from build123d import *

# Parameters (mm, degrees)
SKETCH1_R               = 12.7
EXTRUDE1_DEPTH          = 76.2
SKETCH2_R               = 5
EXTRUDE2_DEPTH          = 2
SKETCH3_R               = 13.7
EXTRUDE3_DEPTH          = 4
SKETCH4_R               = 4
EXTRUDE4_DEPTH          = 7
SKETCH5_W               = 279.527972269
SKETCH5_H               = 9.602426348
CUT_EXTRUDE1_DEPTH      = 14.7
CUT_EXTRUDE1_DEPTH_BACK = 14.7


with BuildPart() as part:
    # Sketch1 → Extrude1 (new body)
    with BuildSketch(Plane(origin=(0, 0, 0), x_dir=(0, 0, -1), z_dir=(1, 0, 0))):
        Circle(SKETCH1_R)
    extrude(amount=EXTRUDE1_DEPTH)

    # Sketch2 → Extrude2 (add, symmetric)
    with BuildSketch(Plane.XY):
        with BuildLine():
            Line((0, 9.805687548), (-19.733094472, 9.805687548))
            ThreePointArc((-19.733094472, 9.805687548), (-29.53878202, 0), (-19.733094472, -9.805687548))
            Line((-19.733094472, -9.805687548), (0, -9.805687548))
            Line((0, -9.805687548), (0, 9.805687548))
        make_face()
        with Locations((-19.733094472, 0)):
            Circle(SKETCH2_R, mode=Mode.SUBTRACT)
    extrude(amount=EXTRUDE2_DEPTH, both=True)

    # Sketch3 → Extrude3 (add)
    with BuildSketch(Plane(origin=(76.2, 0, 0), x_dir=(0, 0, -1), z_dir=(1, 0, 0))):
        Circle(SKETCH3_R)
    extrude(amount=EXTRUDE3_DEPTH)

    # Sketch4 → Extrude4 (add, symmetric)
    with BuildSketch(Plane.XY):
        with BuildLine():
            Line((80.2, 9.635666442), (106.2, 9.635666442))
            ThreePointArc((106.2, 9.635666442), (115.835666442, 0), (106.2, -9.635666442))
            Line((106.2, -9.635666442), (80.2, -9.635666442))
            Line((80.2, -9.635666442), (80.2, 9.635666442))
        make_face()
        with Locations((106.2, 0)):
            Circle(SKETCH4_R, mode=Mode.SUBTRACT)
    extrude(amount=EXTRUDE4_DEPTH, both=True)

    # Sketch5 → Cut-Extrude1 (cut, two sides)
    with BuildSketch(Plane(origin=(0, 0, 0), x_dir=(1, 0, 0), z_dir=(0, 1, 0))) as cut_extrude1_sk:
        with Locations((219.963986135, 0)):
            Rectangle(SKETCH5_W, SKETCH5_H)
    extrude(amount=CUT_EXTRUDE1_DEPTH, mode=Mode.SUBTRACT)
    extrude(cut_extrude1_sk.sketch, amount=-CUT_EXTRUDE1_DEPTH_BACK, mode=Mode.SUBTRACT)


solid = part.part
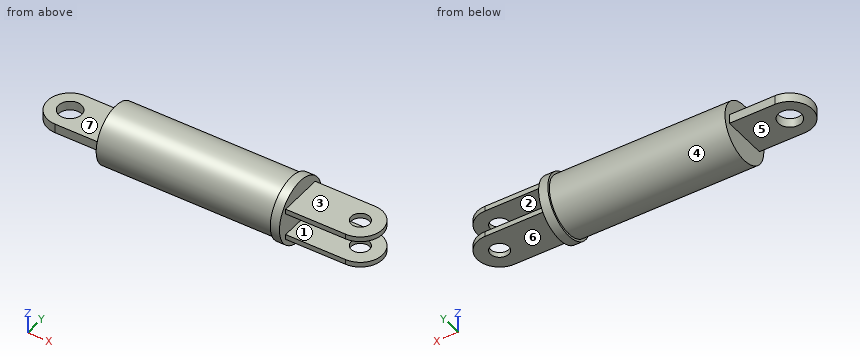
The model under review builds one solid part; all positions refer to its coordinate system, in mm. Face numbers are marked on the shaded views. A direction names the side the tool comes from. Coordinates: 2 decimals unless noted, no trailing zeros. Write each loop counter-clockwise with the first axis right and the second up, starting at its lowest first coordinate (ties: lowest second). Pieces come first, ordered by that corner, then holes. Notation, with made-up numbers: (-20.5, 87) -> (-8.5, 87) arc R31 cw to (-8.5, 123) -> close; hole circle Ø11 at (12, 52.25). An arc over 180 degrees is marked (long way). Answer in a Markdown table with one row per item.
1. Wall thickness on probe 1 along Y at (x, z) = (106.2, -5.75); probe 2 along Z at (x, y) = (99, 0.25); probe 3 along X at (y, z) = (-0.5, -11): over which ranges is each line inside the solid? List them lowest first. Write a range as [from, to].
Answers below:
| item | result |
|---|---|
| probe 1 | y = [-9.64, -4], [4, 9.64] |
| probe 2 | z = [-7, -4.8], [4.8, 7] |
| probe 3 | x = [0, 80.2] |
2. Draft analysis for pull direction Z (two halves, no side actions). For the marked faces 1, 2, 3 and 4, state which applies: +Z half, -Z half, draft (parallel to the pull), parting line (faces both ways), or undercut.
Answers below:
| item | result |
|---|---|
| face 1 | undercut |
| face 2 | undercut |
| face 3 | +Z half |
| face 4 | parting line |
3. We need section A-A, the plane y = 0. Give the number of separate pieces and of enclosed holes in the cut face, and give its area (3 significant figures).
Answers below:
| item | result |
|---|---|
| separate pieces | 4 |
| enclosed holes | 0 |
| area | 2,240 mm^2 |
4. We need section B-B, the plane z = 0. State the section outline as (x, y) points, and give its area (3 significant figures).
Answers below:
| item | result |
|---|---|
| outline | (-19.73, -9.81) -> (0, -9.81) -> (0, -12.7) -> (76.2, -12.7) -> (76.2, -13.7) -> (80.2, -13.7) -> (80.2, 13.7) -> (76.2, 13.7) -> (76.2, 12.7) -> (0, 12.7) -> (0, 9.81) -> (-19.73, 9.81) arc R9.81 ccw to start; hole circle Ø10 at (-19.73, 0) |
| area | 2,500 mm^2 |
5. We need section C-C, the plane x = 93. State the section outline as (y, z) points.
Answers below:
| item | result |
|---|---|
| outline | (-9.64, -7) -> (9.64, -7) -> (9.64, -4.8) -> (-9.64, -4.8) -> close; (-9.64, 4.8) -> (9.64, 4.8) -> (9.64, 7) -> (-9.64, 7) -> close |
6. For the marked faces 5, 6 and 7, list the 3-axis set-ups (+Z, -Z, +X, -X, +Y, -Y) from which the entire face can be reached by the end or side of a thin tool; tool diameter is ignored.
Answers below:
| item | result |
|---|---|
| face 5 | -Z, -X, +Y, -Y |
| face 6 | -Z, +X, +Y, -Y |
| face 7 | +Z, -X, +Y, -Y |
7. Clearance check with flat-ended pins moving along their axes: pin 1 Ø1.5 at (x, y) = (36.5, 0) entering from -Z; pin 2 Ø5 at (x, z) = (41, -9) entering from -Y; pin 3 Ø10 at (x, y) = (-18, 4.5) entering from -Z; pin 4 Ø7 at (x, y) = (106.2, 0) entering from -Z. State where each tip first meets the part, or that it passes through.
Answers below:
| item | result |
|---|---|
| pin 1 | stops at z = -12.7 |
| pin 2 | stops at y = -10.91 |
| pin 3 | stops at z = -2 |
| pin 4 | passes through |
8. We need section D-D, the plane y = -8.25. State the section outline as (x, z) points.
Answers below:
| item | result |
|---|---|
| outline | (-25.03, -2) -> (0, -2) -> (0, -9.66) -> (76.2, -9.66) -> (76.2, -10.94) -> (80.2, -10.94) -> (80.2, -7) -> (111.18, -7) -> (111.18, -4.8) -> (80.2, -4.8) -> (80.2, 4.8) -> (111.18, 4.8) -> (111.18, 7) -> (80.2, 7) -> (80.2, 10.94) -> (76.2, 10.94) -> (76.2, 9.66) -> (0, 9.66) -> (0, 2) -> (-25.03, 2) -> close |
